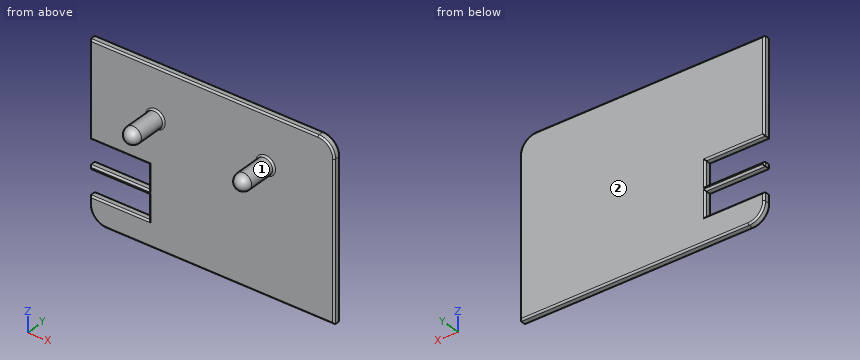
from build123d import *

# Parameters (mm, degrees)
F1_DEPTH = 9
F2_R     = 10
F3_DEPTH = 45
F4_W     = 71.969155259
F4_H     = 30
F5_DEPTH = 25
F6_W     = 71.969155259
F6_H     = 30
F7_DEPTH = 25
F8_R     = 2
F9_R     = 2
F10_R    = 10
F11_R    = 10


with BuildPart() as f1:
    # F0 (on Front) → F1 (new body)
    with BuildSketch(Plane.XZ):
        with BuildLine():
            Line((123.8927025199, 74.8835833272), (-153.1072974801, 74.8835833272))
            Line((-153.1072974801, 74.8835833272), (-153.1072974801, -115.1164166728))
            ThreePointArc((-153.1072974801, -115.1164166728), (-147.2494331038, -129.2585522966), (-133.1072974801, -135.1164166728))
            Line((-133.1072974801, -135.1164166728), (143.8927025199, -135.1164166728))
            Line((143.8927025199, -135.1164166728), (143.8927025199, 54.8835833272))
            ThreePointArc((143.8927025199, 54.8835833272), (138.0348381436, 69.0257189509), (123.8927025199, 74.8835833272))
        make_face()
    extrude(amount=F1_DEPTH)

    # F2 (on face) → F3 (join)
    with BuildSketch(Plane.XZ.offset(9)):
        with Locations((60.3762370774, 14.8835833272)):
            Circle(F2_R)
        with Locations((-73.6063314903, 14.8835833272)):
            Circle(F2_R)
    extrude(amount=F3_DEPTH)

    # F4 (on face) → F5 (cut)
    with BuildSketch(Plane.XZ.offset(9)):
        with Locations((-117.1227198506, -90.1164166728)):
            Rectangle(F4_W, F4_H)
    extrude(amount=-F5_DEPTH, mode=Mode.SUBTRACT)

    # F6 (on face) → F7 (cut)
    with BuildSketch(Plane.XZ.offset(9)):
        with Locations((-117.1227198506, -55.1164166728)):
            Rectangle(F6_W, F6_H)
    extrude(amount=-F7_DEPTH, mode=Mode.SUBTRACT)

    # F8
    f8_edges = [f1.edges().sort_by_distance(p)[0] for p in [
        (143.892703, -9, -40.116417),
        (5.392703, -9, -135.116417),
        (-147.249433, -9, -129.258552),
        (-153.107297, -9, -110.116417),
        (-117.12272, -9, -105.116417),
        (-81.138142, -9, -90.116417),
        (-117.12272, -9, -75.116417),
        (-153.107297, -9, -72.616417),
        (-117.12272, -9, -70.116417),
        (-81.138142, -9, -55.116417),
        (-117.12272, -9, -40.116417),
        (-153.107297, -9, 17.383583),
        (-14.607297, -9, 74.883583),
        (138.034838, -9, 69.025719),
        (-83.606331, -9, 14.883583),
        (50.376237, -9, 14.883583),
    ]]
    fillet(f8_edges, radius=F8_R)

    # F9
    f9_edges = [f1.edges().sort_by_distance(p)[0] for p in [
        (143.892703, 0, -40.116417),
        (5.392703, 0, -135.116417),
        (-147.249433, 0, -129.258552),
        (-153.107297, 0, -110.116417),
        (-117.12272, 0, -105.116417),
        (-81.138142, 0, -90.116417),
        (-117.12272, 0, -75.116417),
        (-153.107297, 0, -72.616417),
        (-117.12272, 0, -70.116417),
        (-81.138142, 0, -55.116417),
        (-117.12272, 0, -40.116417),
        (-153.107297, 0, 17.383583),
        (-14.607297, 0, 74.883583),
        (138.034838, 0, 69.025719),
    ]]
    fillet(f9_edges, radius=F9_R)

    # F10
    f10_edges = [f1.edges().sort_by_distance(p)[0] for p in [
        (-83.606331, -54, 14.883583),
    ]]
    fillet(f10_edges, radius=F10_R)

    # F11
    f11_edges = [f1.edges().sort_by_distance(p)[0] for p in [
        (50.376237, -54, 14.883583),
    ]]
    fillet(f11_edges, radius=F11_R)


solid = f1.part
Work out the finished part from the listing and answer in its coordinate system (mm). Face numbers are marked on the shaded views. Coordinates: 2 decimals unless noted, no trailing zeros. Order: outer loops, then holes, each group sorted by start corner. A loop starts at its lowest first (then second) coordinate and runs counter-clockwise, first axis right, second up. Notation, with made-up numbers: (-14, 81) - (26, 81) arc R30 ccw to (26, 117) - close; hole circle Ø9 at (1, -40). An arc over 180 degrees is marked (long way). Put each result on its own line as item: value. Start each with the question number.
1) Find the intervals of material crossed by line 1 (Y direction, x = -126, z = -38); line 2 (X direction, y = -5.5, z = -103); line 3 (Z direction, x = 16, y = -8.5), in increasing order. Write a range as from..to.
2) For a pull along X with two mould halves and no side action, classify the marked faces 1 and 2 as released by +X, released by -X, zero draft, split by the parting line, or undercut.
3) Find section A-A (z = -47). Give the vertices of the cut face in (x, y), plus the area to 3 significant figures.
4) Find section B-B (x = -14). Give the vertices of the cut face in (y, z).
5) Find section D-D (y = -30). Give the vertices of the cut face in (x, z).
6) Find section C-C (y = -50). Give the vertices of the cut face in (x, z), plus the area to 3 significant figures.
7) Flat-ended cylindrical pins translate along their axes: pin 1 (4 mm diameter, centred on y = -5.5, z = -60.5, fed in from -X); pin 2 (12 mm diameter, centred on x = -63.5, y = -36, fed in from +Z); pin 3 (1 mm diameter, centred on x = -21.5, z = -40.5, fed in from -Y); pin 4 (1 mm diameter, centred on y = -11, z = -102, fed in from +X). Find the tip coordinate at first contact, or state that the pin passes through.
Results list:
1. line 1: y = -9..0
1. line 2: x = -81.14..143.89
1. line 3: z = -134.44..74.21
2. face 1: undercut
2. face 2: zero draft
3. outline: (-81.14, -7) arc R2 ccw to (-79.14, -9) - (141.89, -9) arc R2 ccw to (143.89, -7) - (143.89, -2) arc R2 ccw to (141.89, 0) - (-79.14, 0) arc R2 ccw to (-81.14, -2) - close
3. area: 2,020 mm^2
4. outline: (-9, -133.12) arc R2 ccw to (-7, -135.12) - (-2, -135.12) arc R2 ccw to (0, -133.12) - (0, 72.88) arc R2 ccw to (-2, 74.88) - (-7, 74.88) arc R2 ccw to (-9, 72.88) - close
5. outline: circle Ø20 at (-73.61, 14.88); circle Ø20 at (60.38, 14.88)
6. outline: circle Ø16 at (-73.61, 14.88); circle Ø16 at (60.38, 14.88)
6. area: 402 mm^2
7. pin 1: stops at x = -81.14
7. pin 2: stops at z = 24
7. pin 3: stops at y = -9
7. pin 4: passes through
